from build123d import *

# Parameters (mm, degrees)
F0_W     = 99.06
F0_H     = 71.12
F1_DEPTH = 6.35
F2_W     = 95.377
F2_H     = 63.627
F3_DEPTH = 1.27
F4_W     = 44.577
F4_H     = 12.827
F5_DEPTH = 1.27
F6_W     = 6.35
F6_H     = 6.35
F7_DEPTH = 27.2415


with BuildPart() as f1:
    # F0 (on Top) → F1 (new body)
    with BuildSketch(Plane.XY):
        Rectangle(F0_W, F0_H)
    extrude(amount=F1_DEPTH)

    # F2 (on face) → F3 (cut)
    with BuildSketch(Plane.XY.offset(6.35)):
        Rectangle(F2_W, F2_H)
    extrude(amount=-F3_DEPTH, mode=Mode.SUBTRACT)

    # F4 (on face) → F5 (cut)
    with BuildSketch(Plane.XY.offset(5.08)):
        Rectangle(F4_W, F4_H)
    extrude(amount=-F5_DEPTH, mode=Mode.SUBTRACT)

    # F6 (on face) → F7 (cut, through all)
    with BuildSketch(Plane(origin=(-49.53, 0, 0), x_dir=(0, -1, 0), z_dir=(-1, 0, 0))):
        with Locations((0, 3.175)):
            Rectangle(F6_W, F6_H)
    extrude(amount=-F7_DEPTH, mode=Mode.SUBTRACT)


solid = f1.part
The listing builds one solid part. Answer for the finished solid, in the listing's coordinates (mm). A direction names the side the tool comes from. Coordinates: 2 decimals unless noted, no trailing zeros. Write each loop counter-clockwise with the first axis right and the second up, starting at its lowest first coordinate (ties: lowest second). Pieces come first, ordered by that corner, then holes. Notation, with made-up numbers: M 75.5,87 L 123.5,87 A23 ccw 123.5,118 Z; hole C 32,-2.75 d7. An arc over 180 degrees is marked long. Use one line per item in the form item = value.
Item 1: Find the intervals of material crossed by probe 1 along Y at (x, z) = (-26, 1.5) (3 decimals); probe 2 along X at (y, z) = (14, 6); probe 3 along Y at (x, z) = (4.5, 4.25), in increasing order.
Model answer:
probe_1 = -35.56 to -3.175, 3.175 to 35.56
probe_2 = -49.53 to -47.69, 47.69 to 49.53
probe_3 = -35.56 to -6.41, 6.41 to 35.56
Item 2: Find section B-B, the plane y = -29.5. Give the vertices of the cut face in (x, z), plus the area to 3 significant figures.
Model answer:
outline = M -49.53,0 L 49.53,0 L 49.53,6.35 L 47.69,6.35 L 47.69,5.08 L -47.69,5.08 L -47.69,6.35 L -49.53,6.35 Z
area = 508 mm2
Item 3: Find section D-D, the plane x = -5. Give the vertices of the cut face in (y, z).
Model answer:
outline = M -35.56,0 L 35.56,0 L 35.56,6.35 L 31.81,6.35 L 31.81,5.08 L 6.41,5.08 L 6.41,3.81 L -6.41,3.81 L -6.41,5.08 L -31.81,5.08 L -31.81,6.35 L -35.56,6.35 Z
Item 4: Find section C-C, the plane z = 2.5. Give the vertices of the cut face in (x, y) (1 decimal), plus the area to 3 significant figures.
Model answer:
outline = M -49.5,-35.6 L 49.5,-35.6 L 49.5,35.6 L -49.5,35.6 L -49.5,3.2 L -22.3,3.2 L -22.3,-3.2 L -49.5,-3.2 Z
area = 6,870 mm2
Item 5: For faces 5 (the face through (-22.289, 0, 2)), 6 (the face through (-1, 0, 0)), 7 (the face through (-1, 8, 5.08)), determine the directions among +Z, -Z, +X, -X, +Y, -Y from which every point of the face is accessible in a straight line to the end or side of a thin tool.
Model answer:
face_5 = +Z, -Z, -X
face_6 = -Z, +X, -X, +Y, -Y
face_7 = +Z
Item 6: Given P1, Ø6, axis at x = -23, y = -13.5, coming from the +Z side; P2, Ø0.6, axis at y = -2.5, z = 4.5, coming from the -X side; P3, Ø1.9, axis at y = -1.5, z = 1.5, coming from the -X side, each flat-ended and moving along its own axis, determine where each tip first touches the part or whether it passes through.
Model answer:
P1 = 5.08
P2 = 22.29
P3 = -22.29
Item 7: The mould has two halves that part along X. Classify faces 1 (the face through (-15, -34, 6.35)), 2 (the face through (0, 0, 3.81)), 3 (the face through (49.53, 0, 3)), 4 (the face through (-49.53, -20, 3)): released by +X, released by -X, zero draft, split by the parting line, or undercut.
Model answer:
face_1 = zero draft
face_2 = undercut
face_3 = released by +X
face_4 = released by -X
